The model under review builds one solid part; all positions refer to its coordinate system, in mm. A direction names the side the tool comes from. Round coordinates to 2 decimals unless told otherwise and drop trailing zeros. Order: outer loops, then holes, each group sorted by start corner. A loop starts at its lowest first (then second) coordinate and runs counter-clockwise, first axis right, second up.
from build123d import *

# Parameters (mm, degrees)
SKETCH001_R  = 2
HOLE_DEPTH   = 20.626
CHAMFER_SIZE = 0.25


with BuildPart() as part:
    # Sketch → Revolution (revolve)
    with BuildSketch(Plane.XZ):
        Polygon((0, 2.55), (0, 6.875), (25, 6.875), (25, 4.05), (12.5, 4.05), (12.5, 2.55), align=None)
    revolve(axis=Axis((0, 0, 0), (1, 0, 0)))

    # Sketch001 → Hole (cut, through all)
    with BuildSketch(Plane.XY.offset(13.75)):
        with Locations((5, 0)):
            Circle(SKETCH001_R)
        with Locations((20, 0)):
            Circle(SKETCH001_R)
    extrude(amount=-HOLE_DEPTH, mode=Mode.SUBTRACT)

    # Chamfer
    chamfer_edges = [part.edges().sort_by_distance(p)[0] for p in [
        (25, 0, -6.875),
        (0, 0, -6.875),
        (25, 0, -4.05),
        (0, 0, -2.55),
        (5, 2, 6.577661),
        (5, -2, 6.577661),
        (20, -2, 6.577661),
        (20, 2, 6.577661),
        (3, 0, -6.875),
        (18, 0, -6.875),
    ]]
    chamfer(chamfer_edges, length=CHAMFER_SIZE)


solid = part.part
(1) We need section A-A (z = 0). Give the boundary of the cut face in (x, y) (3 decimals), and give its area (4 significant figures).
(2) To check wall thickness, follow L1, parallel to Y at x = 22, z = 0 (3 decimals); L2, parallel to X at y = 0, z = 5.5; L3, parallel to Z at x = 8.75, y = 0 (3 decimals). State the ranges of each line that lie inside material, in increasing order.
(3) The part is to be moulded in two halves that separate along Z. For faces 1 (the cylindrical face through (18.539, 2.464, -3.214)), 2 (the cylindrical face through (12.67, 2.63, 6.35)), 3 (the cylindrical face through (5.923, -1.774, 4.139)), say which applies: pulls with the +Z half, pulls with the -Z half, needs draft (parallel to the pull), parting line crosses it, or undercut.
(4) We need section C-C (y = -1.5). Count the separate pieces of the cut face and the enclosed holes in it, and give its area (3 significant figures).
(5) We need section B-B (x = 13). Give the boundary of the cut face in (y, z) (3 decimals), and give its area (3 significant figures).
(6) Tool access review of faces 4 (the cylindrical face through (3, 0, -5)), 5 (the flat face through (12.5, 3, 0)): name each direction out of +Z, -Z, +X, -X, +Y, -Y from which nothing blocks a thin tool from reaching the whole face with its end or side.
(7) Clearance check with flat-ended pins moving along their axes: P1, Ø3, axis at y = 0, z = 0, coming from the -X side; P2, Ø1, axis at y = 0.5, z = 2.5, coming from the +X side; P3, Ø4, axis at x = 5.5, z = -2.5, coming from the +Y side; P4, Ø1.5, axis at x = 5, y = -4, coming from the -Z side. State where each tip first meets the part, or that it passes through.
Verdict:
1. outline: (0, -6.625) - (0.25, -6.875) - (24.75, -6.875) - (25, -6.625) - (25, -4.3) - (24.75, -4.05) - (12.5, -4.05) - (12.5, -2.55) - (0.25, -2.55) - (0, -2.8) - close; (0, 2.8) - (0.25, 2.55) - (12.5, 2.55) - (12.5, 4.05) - (24.75, 4.05) - (25, 4.3) - (25, 6.625) - (24.75, 6.875) - (0.25, 6.875) - (0, 6.625) - close
1. area: 178.5 mm2
2. L1: y = -6.875 to -4.05, 4.05 to 6.875
2. L2: x = 0 to 3, 7 to 18, 22 to 25
2. L3: z = -6.875 to -2.55, 2.55 to 6.875
3. face 1: undercut
3. face 2: parting line crosses it
3. face 3: needs draft
4. separate pieces: 6
4. enclosed holes: 0
4. area: 149 mm2
5. outline: circle Ø13.75 at (0, 0); hole circle Ø8.1 at (0, 0)
5. area: 97.0 mm2
6. face 4: +Z, -Z
6. face 5: +X
7. P1: passes through
7. P2: stops at x = 12.5
7. P3: stops at y = 6.86
7. P4: stops at z = -6.06
